Here's how the part is built. I have some questions about the finished solid (model axes, mm). Face numbers are marked on the shaded views. A direction names the side the tool comes from. Give positions to 0.01 mm unless a question says otherwise; leave off trailing zeros. Loops run counter-clockwise (first coordinate to the right, second up) from the corner with the lowest first, then second, coordinate; pieces in that order, holes last. Notation, with made-up numbers: (24.5, 40.25) -> (71.5, 40.25) arc R18 ccw to (71.5, 47.25) -> close; hole circle Ø10 at (80, -17.75). An arc over 180 degrees is marked (long way). Answer in a Markdown table with one row per item. Add a question column.
Item 1: If we section it at A-A (x = -2): Write out the boundary of the cut face in (y, z).
Item 2: If I drill on line 1 (Z direction, x = -16, y = 5.5); line 2 (X direction, y = 3.5, z = -0.25); line 3 (Y direction, x = -11.25, z = 6), over which ranges is the centre line in solid material (lowest first)?
Item 3: If we section it at C-C (y = 8.5): Write out the boundary of the cut face in (x, z).
Item 4: We'd pull the mould along Z, two halves only. Please class the marked faces 1, 2 and 3: released by +Z, released by -Z, zero draft, split by the parting line, or undercut.
Item 5: If we section it at B-B (x = -16): Write out the boundary of the cut face in (y, z).
Item 6: If we section it at D-D (x = -7.5): Write out the boundary of the cut face in (y, z), then the cut area to 3 significant figures.
Item 7: For P1, Ø6, axis at y = 28, z = -6, coming from the -X side; P2, Ø3.5, axis at x = -18.5, y = 20.5, coming from the +Z side; P3, Ø6, axis at x = -16, z = 8, coming from the +Y side; P4, Ø2.5, axis at y = 25, z = 8, coming from the +X side, each with a flat end and sliding along its axis, tell me the tip position at first contact or that it passes through.
Item 8: Which directions (+Z, -Z, +X, -X, +Y, -Y) give clear straight access to the entire face, cutting with the end or side of a thin tool? Please do the marked faces 4, 5 and 6.
```python
from build123d import *

# Parameters (mm, degrees)
BOSS_EXTRUDE1_DEPTH = 14
SKETCH2_R           = 4
CUT_EXTRUDE1_DEPTH  = 44.646305686
SKETCH3_W           = 0.5
SKETCH3_H           = 28
CUT_EXTRUDE2_DEPTH  = 44.646305686
SKETCH4_R           = 2.25
CUT_EXTRUDE3_DEPTH  = 38.536648758
CUT_EXTRUDE4_DEPTH  = 40.56008089
CHAMFER1_SIZE       = 2.5
BOSS_EXTRUDE2_DEPTH = 2.5


with BuildPart() as part:
    # Sketch1 → Boss-Extrude1 (new, symmetric)
    with BuildSketch(Plane.XY):
        Polygon((0, 0), (-22, 0), (-22, 8), (-10, 8), (-10, 35), (0, 35), align=None)
    extrude(amount=BOSS_EXTRUDE1_DEPTH, both=True)

    # Sketch2 → Cut-Extrude1 (cut, through all)
    with BuildSketch(Plane(origin=(0, 35, 0), x_dir=(1, 0, 0), z_dir=(0, 1, 0))):
        Circle(SKETCH2_R)
    extrude(amount=-CUT_EXTRUDE1_DEPTH, mode=Mode.SUBTRACT)

    # Sketch3 → Cut-Extrude2 (cut, through all)
    with BuildSketch(Plane(origin=(0, 35, 0), x_dir=(1, 0, 0), z_dir=(0, 1, 0))):
        with Locations((-0.25, 0)):
            Rectangle(SKETCH3_W, SKETCH3_H)
    extrude(amount=-CUT_EXTRUDE2_DEPTH, mode=Mode.SUBTRACT)

    # Sketch4 → Cut-Extrude3 (cut, through all)
    with BuildSketch(Plane(origin=(0, 8, 0), x_dir=(1, 0, 0), z_dir=(0, 1, 0))):
        with Locations(Location((-16, 8, 0), (0, 0, 180))):
            Circle(SKETCH4_R)
        with Locations(Location((-16, -8, 0), (0, 0, 180))):
            Circle(SKETCH4_R)
    extrude(amount=-CUT_EXTRUDE3_DEPTH, mode=Mode.SUBTRACT)

    # Sketch5 → Cut-Extrude4 (cut, through all)
    with BuildSketch(Plane.ZY.offset(10)):
        with BuildLine():
            Line((6.409009742, 26.590990258), (8, 28.181980515))
            Line((8, 28.181980515), (9.590990258, 26.590990258))
            ThreePointArc((9.590990258, 26.590990258), (8, 22.75), (6.409009742, 26.590990258))
        make_face()
        with BuildLine():
            Line((-9.590990258, 26.590990258), (-8, 28.181980515))
            Line((-8, 28.181980515), (-6.409009742, 26.590990258))
            ThreePointArc((-6.409009742, 26.590990258), (-8, 22.75), (-9.590990258, 26.590990258))
        make_face()
    extrude(amount=-CUT_EXTRUDE4_DEPTH, mode=Mode.SUBTRACT)

    # Chamfer1
    chamfer1_edges = [part.edges().sort_by_distance(p)[0] for p in [
        (-22, 4, 14),
        (-22, 4, -14),
    ]]
    chamfer(chamfer1_edges, length=CHAMFER1_SIZE)

    # Sketch6 → Boss-Extrude2 (add, symmetric)
    with BuildSketch(Plane.XY):
        Polygon((-22, 8), (-22, 14), (-14, 35), (-10, 35), (-10, 8), align=None)
    extrude(amount=BOSS_EXTRUDE2_DEPTH, both=True)


solid = part.part
```
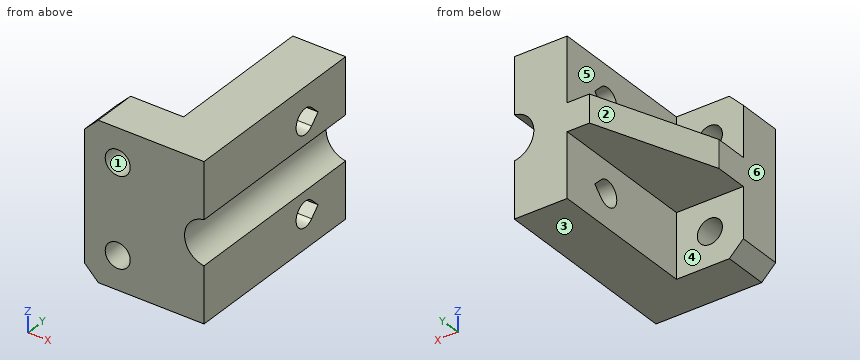
Recorded:
| question | item | result |
|---|---|---|
| 1 | outline | (0, -14) -> (35, -14) -> (35, -3.46) -> (0, -3.46) -> close; (0, 3.46) -> (35, 3.46) -> (35, 14) -> (0, 14) -> close; hole (26.59, -9.59) -> (28.18, -8) -> (26.59, -6.41) arc R2.25 ccw (long way) to start; hole (26.59, 6.41) -> (28.18, 8) -> (26.59, 9.59) arc R2.25 ccw (long way) to start |
| 2 | line 1 | z = -14 to -10.25, -5.75 to 5.75, 10.25 to 14 |
| 2 | line 2 | x = -22 to -3.99 |
| 2 | line 3 | y = 0 to 8 |
| 3 | outline | (-22, -2.5) -> (-10, -2.5) -> (-10, -14) -> (-0.5, -14) -> (-0.5, -3.97) arc R4 cw to (-0.5, 3.97) -> (-0.5, 14) -> (-10, 14) -> (-10, 2.5) -> (-22, 2.5) -> close |
| 4 | face 1 | undercut |
| 4 | face 2 | zero draft |
| 4 | face 3 | released by -Z |
| 5 | outline | (0, -14) -> (8, -14) -> (8, -10.25) -> (0, -10.25) -> close; (0, -5.75) -> (8, -5.75) -> (8, -2.5) -> (29.75, -2.5) -> (29.75, 2.5) -> (8, 2.5) -> (8, 5.75) -> (0, 5.75) -> close; (0, 10.25) -> (8, 10.25) -> (8, 14) -> (0, 14) -> close |
| 6 | outline | (0, -14) -> (35, -14) -> (35, 14) -> (0, 14) -> close; hole (26.59, -9.59) -> (28.18, -8) -> (26.59, -6.41) arc R2.25 ccw (long way) to start; hole (26.59, 6.41) -> (28.18, 8) -> (26.59, 9.59) arc R2.25 ccw (long way) to start |
| 6 | area | 946 mm^2 |
| 7 | P1 | stops at x = -10 |
| 7 | P2 | stops at z = 2.5 |
| 7 | P3 | stops at y = 8 |
| 7 | P4 | passes through |
| 8 | face 4 | -Z, -X, +Y |
| 8 | face 5 | +Z, -X, +Y |
| 8 | face 6 | +Z, -Z, -X, +Y, -Y |
